Could you check a few things on this drawing? It's one solid part, dimensions in mm from its lowest x, y, z. A direction names the side the tool comes from. Round coordinates to 2 decimals unless told otherwise and drop trailing zeros. Loops run counter-clockwise (first coordinate to the right, second up) from the corner with the lowest first, then second, coordinate; pieces in that order, holes last. Notation, with made-up numbers: M 13,68 L 69,68 A24 cw 69,102 Z; hole C 80.5,87 d11. An arc over 180 degrees is marked long. Use a Markdown table: item, result. Add a question column.
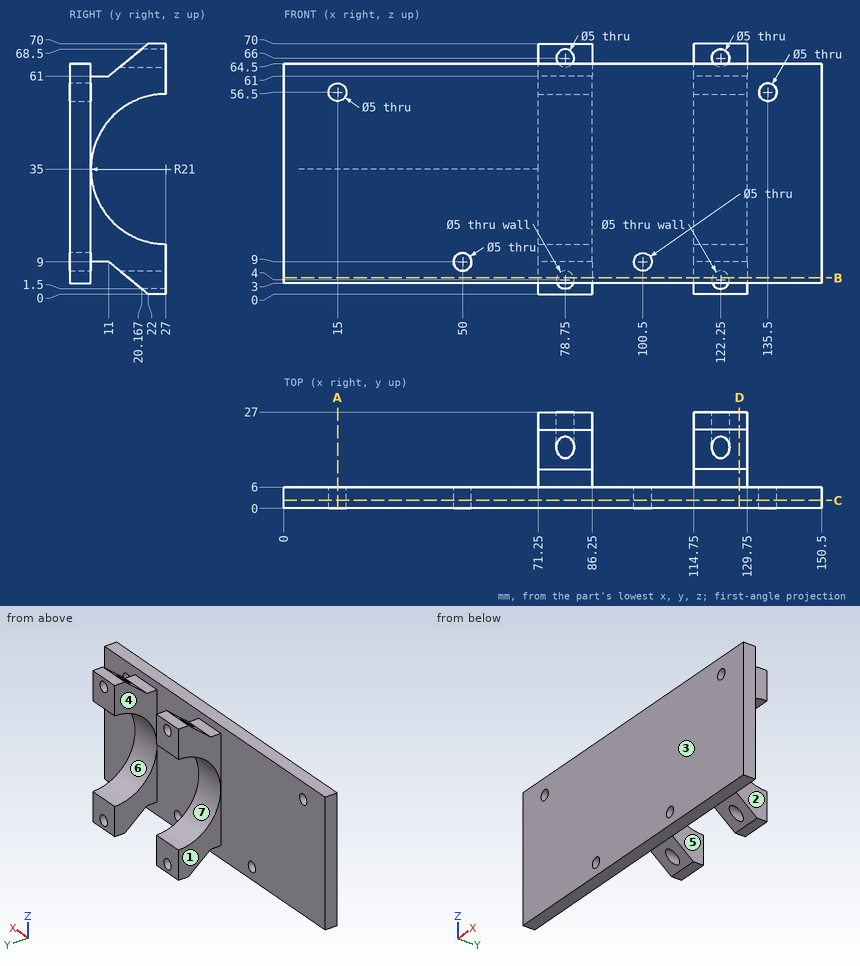
(1) I'm going to push flat-ended pins straight in: pin 1 (6 mm diameter, centred on x = 107.5, z = 35.5, fed in from +Y); pin 2 (4 mm diameter, centred on x = 80.5, y = 10, fed in from -Z); pin 3 (6.5 mm diameter, centred on y = 21.5, z = 17.5, fed in from +X). Where does each tip first touch, or does it pass through?
(2) On a 3-axis mill with a long thin cutter (end or side, diameter ignored), from which of +Z, -Z, +X, -X, +Y, -Y can I reach the whole of each face in a straight line? I mean the marked faces 1, 2, 3 and 4. Say none if no direction works.
(3) Suppose I cut it at D-D on x = 127.5. List the corners of the cut face in (y, z) for me, and give its area (3 significant figures).
(4) Suppose I cut it at A-A on x = 15. List the corners of the cut face in (y, z) for me, and give its area (3 significant figures).
(5) If I drill on probe 1 along X at (y, z) = (3.55, 9); probe 2 along X at (y, z) = (24.25, 4); probe 3 along X at (y, z) = (4.55, 56.5), over which ranges is the centre line in solid material (lowest first)? Write a range as [from, to].
(6) Suppose I cut it at C-C on y = 2.25. List the corners of the cut face in (x, z) for me.
(7) Suppose I cut it at B-B on z = 4.5. List the corners of the cut face in (x, y) for me.
(8) Thinking about a two-plate mould opening in Z: for the marked faces 5, 6 and 7, which applies, released by +Z, released by -Z, zero draft, split by the parting line, or undercut?
Results below:
| question | item | result |
|---|---|---|
| 1 | pin 1 | stops at y = 6 |
| 1 | pin 2 | stops at z = 8.18 |
| 1 | pin 3 | stops at x = 129.75 |
| 2 | face 1 | +Z, -Z, -X, +Y |
| 2 | face 2 | +Z, -Z, +X, +Y |
| 2 | face 3 | +Z, -Z, +X, -X, -Y |
| 2 | face 4 | +Z, -Z, +Y |
| 3 | outline | M 0,3 L 6,3 L 6,9 L 11,9 L 22,0 L 27,0 L 27,14 A21 cw 27,56 L 27,70 L 22,70 L 11,61 L 6,61 L 6,64.5 L 0,64.5 Z |
| 3 | area | 957 mm² |
| 4 | outline | M 0,3 L 6,3 L 6,54 L 0,54 Z; M 0,59 L 6,59 L 6,64.5 L 0,64.5 Z |
| 4 | area | 339 mm² |
| 5 | probe 1 | x = [0, 47.5], [52.5, 98], [103, 150.5] |
| 5 | probe 2 | x = [71.25, 76.25], [81.25, 86.25], [114.75, 119.75], [124.75, 129.75] |
| 5 | probe 3 | x = [0, 12.5], [17.5, 133], [138, 150.5] |
| 6 | outline | M 0,3 L 150.5,3 L 150.5,64.5 L 0,64.5 Z; hole C 15,56.5 d5; hole C 50,9 d5; hole C 100.5,9 d5; hole C 135.5,56.5 d5 |
| 7 | outline | M 0,0 L 150.5,0 L 150.5,6 L 0,6 Z; M 71.25,16.5 L 76.3,16.5 L 76.3,27 L 71.25,27 Z; M 81.2,16.5 L 86.25,16.5 L 86.25,27 L 81.2,27 Z; M 114.75,16.5 L 119.8,16.5 L 119.8,27 L 114.75,27 Z; M 124.7,16.5 L 129.75,16.5 L 129.75,27 L 124.7,27 Z |
| 8 | face 5 | zero draft |
| 8 | face 6 | undercut |
| 8 | face 7 | undercut |
